```python
from build123d import *

# Parameters (mm, degrees)
SKETCH_5_R = 0.3


with BuildPart() as part:
    # Эскиз3 → Повернуть2 (revolve)
    with BuildSketch(Plane.XY):
        with BuildLine():
            Line((0, 0), (-3.25, 0))
            Line((-3.25, 0), (-3.25, 0.3))
            add(Edge.make_bspline(
                [(-2.000000082, 1.199999952), (-2.23604302, 1.181615986), (-2.789263679, 1.00505202), (-2.971144892, 0.430097598), (-3.25, 0.3)],
                knots=[0.780397484, 0.780397484, 0.780397484, 0.780397484, 0.876745066, 1, 1, 1, 1], degree=3))
            add(Edge.make_bspline(
                [(-1.6, 1.180025241), (-1.731399218, 1.201650855), (-1.864601443, 1.21054538), (-2.000000082, 1.199999952)],
                knots=[0.725130753, 0.725130753, 0.725130753, 0.725130753, 0.780397484, 0.780397484, 0.780397484, 0.780397484], degree=3))
            add(Edge.make_bspline(
                [(-1.3, 1.111050082), (-1.34982276, 1.125028982), (-1.449295193, 1.15139314), (-1.549743584, 1.171754066), (-1.6, 1.180025241)],
                knots=[0.682659096, 0.682659096, 0.682659096, 0.682659096, 0.70399282, 0.725130753, 0.725130753, 0.725130753, 0.725130753], degree=3))
            add(Edge.make_bspline(
                [(-0.9, 0.997661651), (-1.033638838, 1.030728014), (-1.166305516, 1.073539075), (-1.3, 1.111050082)],
                knots=[0.62541214, 0.62541214, 0.62541214, 0.62541214, 0.682659096, 0.682659096, 0.682659096, 0.682659096], degree=3))
            add(Edge.make_bspline(
                [(-0.6, 0.946228082), (-0.616698211, 0.947554212), (-0.71755748, 0.957111909), (-0.817198443, 0.977173996), (-0.9, 0.997661651)],
                knots=[0.582920397, 0.582920397, 0.582920397, 0.582920397, 0.589942383, 0.62541214, 0.62541214, 0.62541214, 0.62541214], degree=3))
            add(Edge.make_bspline(
                [(-0.2, 0.945686937), (-0.334396136, 0.941079864), (-0.468154451, 0.935757238), (-0.6, 0.946228082)],
                knots=[0.527476276, 0.527476276, 0.527476276, 0.527476276, 0.582920397, 0.582920397, 0.582920397, 0.582920397], degree=3))
            add(Edge.make_bspline(
                [(0, 0.95), (-0.066719861, 0.950074874), (-0.133438155, 0.947968664), (-0.2, 0.945686937)],
                knots=[0.500016684, 0.500016684, 0.500016684, 0.500016684, 0.527476276, 0.527476276, 0.527476276, 0.527476276], degree=3))
            add(Edge.make_bspline(
                [(0, 0.95), (0.066719861, 0.950074874), (0.133438155, 0.947968664), (0.2, 0.945686937)],
                knots=[0.500016684, 0.500016684, 0.500016684, 0.500016684, 0.527476276, 0.527476276, 0.527476276, 0.527476276], degree=3))
            add(Edge.make_bspline(
                [(0.2, 0.945686937), (0.334396136, 0.941079864), (0.468154451, 0.935757238), (0.6, 0.946228082)],
                knots=[0.527476276, 0.527476276, 0.527476276, 0.527476276, 0.582920397, 0.582920397, 0.582920397, 0.582920397], degree=3))
            add(Edge.make_bspline(
                [(0.6, 0.946228082), (0.616698211, 0.947554212), (0.71755748, 0.957111909), (0.817198443, 0.977173996), (0.9, 0.997661651)],
                knots=[0.582920397, 0.582920397, 0.582920397, 0.582920397, 0.589942383, 0.62541214, 0.62541214, 0.62541214, 0.62541214], degree=3))
            add(Edge.make_bspline(
                [(0.9, 0.997661651), (1.033638838, 1.030728014), (1.166305516, 1.073539075), (1.3, 1.111050082)],
                knots=[0.62541214, 0.62541214, 0.62541214, 0.62541214, 0.682659096, 0.682659096, 0.682659096, 0.682659096], degree=3))
            add(Edge.make_bspline(
                [(1.3, 1.111050082), (1.34982276, 1.125028982), (1.449295193, 1.15139314), (1.549743584, 1.171754066), (1.6, 1.180025241)],
                knots=[0.682659096, 0.682659096, 0.682659096, 0.682659096, 0.70399282, 0.725130753, 0.725130753, 0.725130753, 0.725130753], degree=3))
            add(Edge.make_bspline(
                [(1.6, 1.180025241), (1.731399218, 1.201650855), (1.864601443, 1.21054538), (2, 1.2)],
                knots=[0.725130753, 0.725130753, 0.725130753, 0.725130753, 0.780397484, 0.780397484, 0.780397484, 0.780397484], degree=3))
            add(Edge.make_bspline(
                [(2, 1.2), (2.23604302, 1.181615986), (2.789263679, 1.00505202), (2.971144892, 0.430097598), (3.25, 0.3)],
                knots=[0.780397484, 0.780397484, 0.780397484, 0.780397484, 0.876745066, 1, 1, 1, 1], degree=3))
            Line((3.25, 0.3), (3.25, 0))
            Line((3.25, 0), (0, 0))
        make_face()
    revolve(axis=Axis((0, 0, 0), (1, 0, 0)))

    # По траектории2: sweep along a path in Эскиз4
    with BuildLine(Plane.XY) as sweep_2_path:
        Line((2.987274619, 0), (3.31, 0))
        ThreePointArc((3.31, 0), (3.663553391, -0.146446609), (3.81, -0.5))
        Line((3.81, -0.5), (3.81, -4))
    # Эскиз5 → По траектории2 (sweep)
    with BuildSketch(Plane(origin=(0, -4, 0), x_dir=(1, 0, 0), z_dir=(0, 1, 0))):
        with Locations((3.81, 0)):
            Circle(SKETCH_5_R)
    sweep_2 = sweep(path=sweep_2_path.line)

    # Зеркальное отражение1: По траектории2 across plane
    add(sweep_2.mirror(Plane(origin=(0, 0, 0), x_dir=(0, 0, 1), z_dir=(1, 0, 0))))


solid = part.part
```
Verification items for the finished model (mm, model axes). Coordinates: 2 decimals unless noted, no trailing zeros. Order: outer loops, then holes, each group sorted by start corner. A loop starts at its lowest first (then second) coordinate and runs counter-clockwise, first axis right, second up. Notation, with made-up numbers: (43, 6.5) - (53, 6.5) arc R13 ccw to (53, 22.5) - close; hole circle Ø4 at (33.5, -14). An arc over 180 degrees is marked (long way). Return JSON: item names as keys, results as strings.
(1) Thickness scan on line 1 along Y through (x, z) = (-1.5, -0.3); line 2 along Y through (x, z) = (3, -0.35); line 3 along X through (y, z) = (-2.05, -0.2). Record the ranges inside material, lowest first.
Filled sheet:
{"line 1": "y = -1.12 to 1.12", "line 2": "y = -0.36 to 0.36", "line 3": "x = -4.03 to -3.59, 3.59 to 4.03"}
(2) Section check A-A, the plane y = -3.5. Record the cut outline in (x, z), and give its area (3 significant figures).
Filled sheet:
{"outline": "circle Ø0.6 at (-3.81, 0); circle Ø0.6 at (3.81, 0)", "area": "0.565 mm^2"}
(3) Go/stop test with a flat-tipped pin: pin 1 (1.5 mm diameter, centred on x = 0.5, y = 0.5, fed in from +Z). Record where the tip stops, or that it passes through.
Filled sheet:
{"pin 1": "stops at z = 1.06"}
